```python
from build123d import *

# Parameters (mm, degrees)
SKETCH_R           = 93
PAD_DEPTH          = 1.6
POCKET_DEPTH       = 527.6981773351
POLARPATTERN_COUNT = 4
SKETCH003_R        = 8
POCKET001_DEPTH    = 1.601
SKETCH001_R        = 8
PAD001_DEPTH       = 6
CHAMFER002_SIZE2   = 0.2
CHAMFER002_SIZE    = 3
CHAMFER_SIZE       = 0.8


with BuildPart() as part:
    # Sketch → Pad (new body)
    with BuildSketch(Plane.XY):
        Circle(SKETCH_R)
    extrude(amount=PAD_DEPTH)

    # Sketch002 → Pocket (cut, through all)
    with BuildSketch(Plane.XY):
        with BuildLine():
            Line((-29.7321374946, 4), (-84.9058301885, 4))
            ThreePointArc((-62.8659154133, 57.2090611638), (-78.5297602635, 32.528091751), (-84.9058301885, 4))
            Line((-62.8659154133, 57.2090611638), (-23.8522231664, 18.1953689169))
            ThreePointArc((-23.8522231664, 18.1953689169), (-27.7163859753, 11.480502971), (-29.7321374946, 4))
        make_face()
        with BuildLine():
            Line((-18.1953689169, 23.8522231664), (-57.2090611638, 62.8659154133))
            ThreePointArc((-4, 84.9058301885), (-32.528091751, 78.5297602635), (-57.2090611638, 62.8659154133))
            Line((-4, 29.7321374946), (-4, 84.9058301885))
            ThreePointArc((-4, 29.7321374946), (-11.480502971, 27.7163859753), (-18.1953689169, 23.8522231664))
        make_face()
    pocket = extrude(amount=POCKET_DEPTH, mode=Mode.SUBTRACT)

    # PolarPattern: Pocket ×4 about axis
    polarpattern_axis = Axis((0, 0, 0), (0, 0, 1))
    for i in range(1, POLARPATTERN_COUNT):
        add(pocket.rotate(polarpattern_axis, i * 360 / POLARPATTERN_COUNT), mode=Mode.SUBTRACT)

    # Sketch003 → Pocket001 (cut, through all)
    with BuildSketch(Plane.XY.offset(1.6)):
        Circle(SKETCH003_R)
    extrude(amount=-POCKET001_DEPTH, mode=Mode.SUBTRACT)

    # Sketch001 → Pad001 (join)
    with BuildSketch(Plane.XY.offset(1.6)):
        with BuildLine():
            ThreePointArc((-23.4, 0), (0, -23.4), (23.4, 0))
            ThreePointArc((23.9970767333, 0), (23.6985383667, 0.2704222444), (23.4, 0))
            ThreePointArc((17.6776695297, -17.6776695297), (22.8235419267, -9.5488497004), (23.9970767333, 0))
            ThreePointArc((-25, 0), (-9.5670858091, -23.0969883128), (17.6776695297, -17.6776695297))
            ThreePointArc((19.8, 0), (-2.6, 22.4), (-25, 0))
            ThreePointArc((-9.6, 6e-10), (5.0999999997, -14.7000000003), (19.8, 0))
            ThreePointArc((-5.2392156863, -8.0442910808), (8.4396821797, 4.5751245563), (-9.6, 0))
            ThreePointArc((-5.2392156863, -8.0442910808), (9.3524272192, -12.3905957381), (18.2, 0))
            ThreePointArc((18.2, 0), (-2.6, 20.8), (-23.4, 0))
        make_face()
        Circle(SKETCH001_R, mode=Mode.SUBTRACT)
        with BuildLine():
            ThreePointArc((-11.5, 0), (-16.5, 5), (-21.5, 0))
            ThreePointArc((-21.5, 0), (-5.3119919625, -20.8334524597), (18.8751387339, -10.2946169319))
            ThreePointArc((18.8751387339, -10.2946169319), (18.7741114914, -9.8986944388), (18.3719108937, -9.9707763607))
            ThreePointArc((-11.5, 0), (-0.1557720255, -15.746010937), (18.3719108937, -9.9707763607))
        make_face()
    extrude(amount=PAD001_DEPTH)

    # Chamfer002
    chamfer002_edges = [part.edges().sort_by_distance(p)[0] for p in [
        (-5.311992, -20.833452, 7.6),
    ]]
    chamfer002_side = part.faces().sort_by_distance((-5.311992, -20.833452, 4.6))[0]
    chamfer(chamfer002_edges, length=CHAMFER002_SIZE, length2=CHAMFER002_SIZE2, reference=chamfer002_side)

    # Chamfer
    chamfer_edges = [part.edges().sort_by_distance(p)[0] for p in [
        (-8, 0, 7.6),
    ]]
    chamfer(chamfer_edges, length=CHAMFER_SIZE)


solid = part.part
```
The listing builds one solid part. Answer for the finished solid, in the listing's coordinates (mm). A direction names the side the tool comes from. Round coordinates to 2 decimals unless told otherwise and drop trailing zeros. Write each loop counter-clockwise with the first axis right and the second up, starting at its lowest first coordinate (ties: lowest second). Pieces come first, ordered by that corner, then holes. Notation, with made-up numbers: (89.5, 77.25) -> (99.5, 77.25) arc R31 ccw to (99.5, 108.25) -> close; hole circle Ø2 at (-4.5, -0.5). An arc over 180 degrees is marked (long way). Use CSV: the item, a comma, the result in double quotes. Start each with the question number.
(1) Which of the six approach directions +Z, -Z, +X, -X, +Y, -Y give full straight-line access (tool end or side, diameter ignored) to faces 1 (the face through (-9.947, -22.936, 4.558)), 2 (the face through (-16.4, 5, 3.1)), 3 (the face through (-11.581, -27.675, 0.789))?
(2) Section B-B on z = 2.75 is taken. Give the vertices of the cut face in (x, y), then the cut area to 3 significant figures.
(3) Section C-C on y = -42 is taken. Give the vertices of the cut face in (x, z).
(4) Consider L1, parallel to Y at x = 0, z = 1; L2, parallel to Y at x = 0, z = 5.5; L3, parallel to Z at x = -75.5, y = 44.5. Determine where each line is inside the solid, lowest interval first. Write a range as from..to.
(5) Section A-A on x = -49.5 is taken. Give the vertices of the cut face in (y, z).
(6) Each of these flat-tipped pins is pushed along its axis until it touches: pin 1 (1.3 mm diameter, centred on x = -50.5, z = 0.5, fed in from -Y); pin 2 (1.8 mm diameter, centred on x = 46.5, z = 1, fed in from +Y); pin 3 (1.8 mm diameter, centred on y = -62.5, z = 1, fed in from +X); pin 4 (14.5 mm diameter, centred on x = 0, y = 0, fed in from +Z). Where does it stop, or does it pass through?
(7) Section D-D on y = -65 is taken. Give the vertices of the cut face in (x, z).
(8) The mould has two halves that part along Y. Classify faces 4 (the face through (-5.7, -20.73, 3.08)), 5 (the face through (7, -6, 7.6)), 6 (the face through (-2.107, 22.395, 4.558)), 7 (the face through (88.705, 27.935, 0.789)): released by +Y, released by -Y, zero draft, split by the parting line, or undercut.
A:
1,face 1,"+Z, -Y"
1,face 2,"+Z"
1,face 3,"+Z, -Z"
2,outline,"(-25, 0) arc R25 ccw to (17.68, -17.68) arc R21.94 ccw to (24, 0) arc R0.3 ccw to (23.4, 0) arc R23.4 cw to (-23.4, 0) arc R20.8 cw to (18.2, 0) arc R13.1 cw to (-5.24, -8.04) arc R9.6 ccw (long way) to (-9.6, 0) arc R14.7 ccw to (19.8, 0) arc R22.4 ccw to start; (-21.5, 0) arc R21.5 ccw to (18.88, -10.29) arc R0.3 ccw to (18.37, -9.97) arc R16.6 cw to (-11.5, 0) arc R5 ccw to start; hole circle Ø16 at (0, 0)"
2,area,"704 mm²"
3,outline,"(-82.98, 0) -> (-73.9, 0) -> (-73.9, 1.6) -> (-82.98, 1.6) -> close; (-47.66, 0) -> (-36.34, 0) -> (-36.34, 1.6) -> (-47.66, 1.6) -> close; (-4, 0) -> (4, 0) -> (4, 1.6) -> (-4, 1.6) -> close; (36.34, 0) -> (47.66, 0) -> (47.66, 1.6) -> (36.34, 1.6) -> close; (73.9, 0) -> (82.98, 0) -> (82.98, 1.6) -> (73.9, 1.6) -> close"
4,L1,"y = -93..-8, 8..93"
4,L2,"y = -25..-23.4, -21.44..-15.86, -13.79..-12.07, -9.6..-8, 8..9.6, 20.64..22.25"
4,L3,"z = 0..1.6"
5,outline,"(-78.73, 0) -> (-69.1, 0) -> (-69.1, 1.6) -> (-78.73, 1.6) -> close; (-55.16, 0) -> (-43.84, 0) -> (-43.84, 1.6) -> (-55.16, 1.6) -> close; (-4, 0) -> (4, 0) -> (4, 1.6) -> (-4, 1.6) -> close; (43.84, 0) -> (55.16, 0) -> (55.16, 1.6) -> (43.84, 1.6) -> close; (69.1, 0) -> (78.73, 0) -> (78.73, 1.6) -> (69.1, 1.6) -> close"
6,pin 1,"stops at y = -78.51"
6,pin 2,"stops at y = 81.05"
6,pin 3,"stops at x = 69.67"
6,pin 4,"passes through"
7,outline,"(-66.51, 0) -> (-54.77, 0) -> (-54.77, 1.6) -> (-66.51, 1.6) -> close; (-4, 0) -> (4, 0) -> (4, 1.6) -> (-4, 1.6) -> close; (54.77, 0) -> (66.51, 0) -> (66.51, 1.6) -> (54.77, 1.6) -> close"
8,face 4,"undercut"
8,face 5,"zero draft"
8,face 6,"released by +Y"
8,face 7,"split by the parting line"
